Read the model definition and answer for the solid it produces. Units are mm, in the model's axes. A direction names the side the tool comes from. Round coordinates to 2 decimals unless told otherwise and drop trailing zeros. Order: outer loops, then holes, each group sorted by start corner. A loop starts at its lowest first (then second) coordinate and runs counter-clockwise, first axis right, second up. Notation, with made-up numbers: (-13.75, 3.5) - (42.25, 3.5) arc R20 ccw to (42.25, 41.5) - close; hole circle Ø7 at (61, 30.5). An arc over 180 degrees is marked (long way). Answer as a JSON object with one key per item and string values. Group by question number.
Q1. Consider line 1 (Z direction, x = -10.5, y = 1.4); line 2 (Z direction, x = 32, y = 1.7); line 3 (X direction, y = 0.8, z = 26.5). Determine where each line is inside the solid, lowest interval first.
Q2. A cutting plane is placed at B-B on x = 1. Determine the outline of the cut face in (y, z) (3 decimals), and give its area (3 significant figures).
Q3. A tool of negligible diameter and unlimited length cuts with its end or side. For faces 5 (the flat face through (32.84, -0.03, -19.32)), 6 (the flat face through (30.94, -0.03, -17.53)), from which of +Z, -Z, +X, -X, +Y, -Y can it reach the whole face along a straight path? Write none if from no direction.
Q4. Given pin 1 Ø1 at (y, z) = (0.5, -21.5) entering from +X; pin 2 Ø1 at (y, z) = (1.5, 20.5) entering from -X, each flat-ended and moving along its own axis, determine where each tip first touches the part or whether it passes through.
Q5. A cutting plane is placed at C-C on z = -5.5. Determine the outline of the cut face in (x, y) (3 decimals), and give its area (3 significant figures).
Q6. The mould has two halves that part along X. Classify faces 1 (the flat face through (-30.94, -0.03, 17.53)), 2 (the flat face through (-30.65, -0.03, -18.03)), 3 (the flat face through (33.15, -0.03, 18.78)), 4 (the flat face through (32, 1.905, 17)): pulls with the +X half, pulls with the -X half, needs draft (parallel to the pull), parting line crosses it, or undercut.
Q7. A cutting plane is placed at A-A on y = -0.1. Determine the outline of the cut face in (x, z).
```python
from build123d import *

# Parameters (mm, degrees)
F1_DEPTH = 1.905


with BuildPart() as f1:
    # F0 (on Front) → F1 (new body, symmetric)
    with BuildSketch(Plane.XZ):
        Polygon((-21.997045, -38.1), (21.997045, -38.1), (43.994091, 0), (21.997045, 38.1), (-21.997045, 38.1), (-43.994091, 0), align=None)
        Polygon((-41.061151, 0), (-20.530576, 35.56), (20.530576, 35.56), (41.061151, 0), (20.530576, -35.56), (-20.530576, -35.56), align=None, mode=Mode.SUBTRACT)
    extrude(amount=F1_DEPTH, both=True)


solid = f1.part
```
Result set:
{
 "1": {"line 1": "z = -38.1 to -35.56, 35.56 to 38.1", "line 2": "z = -20.77 to -15.69, 15.69 to 20.77", "line 3": "x = -28.69 to -25.76, 25.76 to 28.69"},
 "2": {"outline": "(-1.905, -38.1) - (1.905, -38.1) - (1.905, -35.56) - (-1.905, -35.56) - close; (-1.905, 35.56) - (1.905, 35.56) - (1.905, 38.1) - (-1.905, 38.1) - close", "area": "19.4 mm²"},
 "3": {"face 5": "-Z, +X, +Y, -Y", "face 6": "+Y, -Y"},
 "4": {"pin 1": "stops at x = 31.87", "pin 2": "stops at x = -32.45"},
 "5": {"outline": "(-40.819, -1.905) - (-37.886, -1.905) - (-37.886, 1.905) - (-40.819, 1.905) - close; (37.886, -1.905) - (40.819, -1.905) - (40.819, 1.905) - (37.886, 1.905) - close", "area": "22.3 mm²"},
 "6": {"face 1": "undercut", "face 2": "undercut", "face 3": "pulls with the +X half", "face 4": "needs draft"},
 "7": {"outline": "(-43.99, 0) - (-22, -38.1) - (22, -38.1) - (43.99, 0) - (22, 38.1) - (-22, 38.1) - close; hole (-41.06, 0) - (-20.53, -35.56) - (20.53, -35.56) - (41.06, 0) - (20.53, 35.56) - (-20.53, 35.56) - close"}
}
